The model under review builds one solid part; all positions refer to its coordinate system, in mm. A direction names the side the tool comes from. Give positions to 0.01 mm unless a question says otherwise; leave off trailing zeros. Order: outer loops, then holes, each group sorted by start corner. A loop starts at its lowest first (then second) coordinate and runs counter-clockwise, first axis right, second up. Notation, with made-up numbers: (55, 59) - (88, 59) arc R28 cw to (88, 79) - close; hole circle Ø5 at (-26.5, 32.25). An arc over 180 degrees is marked (long way). Write item = value, one per line. Start each with the question number.
1. Wall thickness on probe 1 along X at (y, z) = (-14, 125.5); probe 2 along X at (y, z) = (4, 54): over which ranges is each line inside the solid? List them lowest first.
2. Mouldability with a two-part tool opening along X and no side actions: class faces 1 (the flat face through (11, -20, 76)), 2 (the cylindrical face through (-18.717, 18.647, 75.922)), 3 (the flat face through (-7.1, -8.6, 75.9)) as pulls with the +X half, pulls with the -X half, needs draft (parallel to the pull), parting line crosses it, or undercut.
3. Machinability: for faces 4 (the flat face through (-5.385, -17, 76)), 5 (the flat face through (5.385, 17, 76)), 6 (the flat face through (17, 2.966, 76)), 7 (the flat face through (-17, 5.266, 76)), which of the approach directions +Z, -Z, +X, -X, +Y, -Y give a long, thin tool a straight path to every point of the face, cutting with its end or side? Answer none if there is none.
4. We need section B-B, the plane x = 1.5. Give the boundary of the cut face in (y, z), and give its area (3 significant figures).
5. For P1, Ø0.5, axis at x = -6, z = 71.5, coming from the -Y side; P2, Ø1.3, axis at x = -17, z = 62, coming from the -Y side; P3, Ø6, axis at x = -3, z = 45, coming from the +Y side; P4, Ø4, axis at x = 15, y = -14, coming from the -Z side, all flat-tipped, find the tip position at first contact; note any pin that passes through.
6. We need section A-A, the plane y = -7. Give the boundary of the cut face in (x, z).
7. We need section C-C, the plane z = 14. State how many separate pieces and enclosed holes the cut face has, and give its area (3 significant figures).
from build123d import *

# Parameters (mm, degrees)
BOSS_EXTRUDE1_DEPTH  = 154
MIRROR3_COPY_1_DEPTH = 154
MIRROR3_COPY_2_DEPTH = 154


with BuildPart() as part:
    # Sketch1 → Boss-Extrude1 (new body)
    with BuildSketch(Plane.XY):
        with BuildLine():
            Line((3.4, 0), (5.5, 0))
            Line((5.5, 0), (5.5, 4))
            Line((5.5, 4), (11.69, 10.19))
            Line((11.69, 10.19), (18.2, 10.19))
            Line((18.2, 10.19), (18.2, 5.265595036))
            Line((18.2, 5.265595036), (15.5, 5.265595036))
            Line((15.5, 5.265595036), (15.5, 2.965595036))
            Line((15.5, 2.965595036), (19, 2.965595036))
            Line((19, 2.965595036), (19, 3.965595036))
            Line((19, 3.965595036), (20, 3.965595036))
            Line((20, 3.965595036), (20, 15.5))
            ThreePointArc((20, 15.5), (18.681980515, 18.681980515), (15.5, 20))
            Line((15.5, 20), (6.385304712, 20))
            Line((6.385304712, 20), (6.385304712, 19))
            Line((6.385304712, 19), (5.385304712, 19))
            Line((5.385304712, 19), (5.385304712, 15.5))
            Line((5.385304712, 15.5), (7.685304712, 15.5))
            Line((7.685304712, 15.5), (7.685304712, 18.2))
            Line((7.685304712, 18.2), (10.19, 18.2))
            Line((10.19, 18.2), (10.19, 11.69))
            Line((10.19, 11.69), (4, 5.5))
            Line((4, 5.5), (0, 5.5))
            Line((0, 5.5), (0, 3.4))
            ThreePointArc((0, 3.4), (2.404163056, 2.404163056), (3.4, 0))
        make_face()
        with BuildLine():
            Line((18.5, 11.69), (18.5, 15.5))
            ThreePointArc((18.5, 15.5), (17.621320344, 17.621320344), (15.5, 18.5))
            Line((15.5, 18.5), (11.69, 18.5))
            Line((11.69, 18.5), (11.69, 11.69))
            Line((11.69, 11.69), (18.5, 11.69))
        make_face(mode=Mode.SUBTRACT)
    boss_extrude1 = extrude(amount=BOSS_EXTRUDE1_DEPTH)

    # Mirror1: Boss-Extrude1 across plane
    add(boss_extrude1.mirror(Plane.ZX))

    # Mirror2: Boss-Extrude1 across plane
    add(boss_extrude1.mirror(Plane(origin=(0, 0, 0), x_dir=(0, 0, 1), z_dir=(1, 0, 0))))

    # Mirror3 copy 1 sketch → Mirror3 copy 1 (add)
    with BuildSketch(Plane(origin=(0, 0, 0), x_dir=(-1, 0, 0), z_dir=(0, 0, 1))):
        with BuildLine():
            Line((3.4, 0), (5.5, 0))
            Line((5.5, 0), (5.5, 4))
            Line((5.5, 4), (11.69, 10.19))
            Line((11.69, 10.19), (18.2, 10.19))
            Line((18.2, 10.19), (18.2, 5.265595036))
            Line((18.2, 5.265595036), (15.5, 5.265595036))
            Line((15.5, 5.265595036), (15.5, 2.965595036))
            Line((15.5, 2.965595036), (19, 2.965595036))
            Line((19, 2.965595036), (19, 3.965595036))
            Line((19, 3.965595036), (20, 3.965595036))
            Line((20, 3.965595036), (20, 15.5))
            ThreePointArc((20, 15.5), (18.681980515, 18.681980515), (15.5, 20))
            Line((15.5, 20), (6.385304712, 20))
            Line((6.385304712, 20), (6.385304712, 19))
            Line((6.385304712, 19), (5.385304712, 19))
            Line((5.385304712, 19), (5.385304712, 15.5))
            Line((5.385304712, 15.5), (7.685304712, 15.5))
            Line((7.685304712, 15.5), (7.685304712, 18.2))
            Line((7.685304712, 18.2), (10.19, 18.2))
            Line((10.19, 18.2), (10.19, 11.69))
            Line((10.19, 11.69), (4, 5.5))
            Line((4, 5.5), (0, 5.5))
            Line((0, 5.5), (0, 3.4))
            ThreePointArc((0, 3.4), (2.404163056, 2.404163056), (3.4, 0))
        make_face()
        with BuildLine():
            Line((18.5, 11.69), (18.5, 15.5))
            ThreePointArc((18.5, 15.5), (17.621320344, 17.621320344), (15.5, 18.5))
            Line((15.5, 18.5), (11.69, 18.5))
            Line((11.69, 18.5), (11.69, 11.69))
            Line((11.69, 11.69), (18.5, 11.69))
        make_face(mode=Mode.SUBTRACT)
    extrude(amount=MIRROR3_COPY_1_DEPTH)

    # Mirror3 copy 2 sketch → Mirror3 copy 2 (add)
    with BuildSketch(Plane.XY):
        with BuildLine():
            Line((3.4, 0), (5.5, 0))
            Line((5.5, 0), (5.5, -4))
            Line((5.5, -4), (11.69, -10.19))
            Line((11.69, -10.19), (18.2, -10.19))
            Line((18.2, -10.19), (18.2, -5.265595036))
            Line((18.2, -5.265595036), (15.5, -5.265595036))
            Line((15.5, -5.265595036), (15.5, -2.965595036))
            Line((15.5, -2.965595036), (19, -2.965595036))
            Line((19, -2.965595036), (19, -3.965595036))
            Line((19, -3.965595036), (20, -3.965595036))
            Line((20, -3.965595036), (20, -15.5))
            ThreePointArc((20, -15.5), (18.681980515, -18.681980515), (15.5, -20))
            Line((15.5, -20), (6.385304712, -20))
            Line((6.385304712, -20), (6.385304712, -19))
            Line((6.385304712, -19), (5.385304712, -19))
            Line((5.385304712, -19), (5.385304712, -15.5))
            Line((5.385304712, -15.5), (7.685304712, -15.5))
            Line((7.685304712, -15.5), (7.685304712, -18.2))
            Line((7.685304712, -18.2), (10.19, -18.2))
            Line((10.19, -18.2), (10.19, -11.69))
            Line((10.19, -11.69), (4, -5.5))
            Line((4, -5.5), (0, -5.5))
            Line((0, -5.5), (0, -3.4))
            ThreePointArc((0, -3.4), (2.404163056, -2.404163056), (3.4, 0))
        make_face()
        with BuildLine():
            Line((18.5, -11.69), (18.5, -15.5))
            ThreePointArc((18.5, -15.5), (17.621320344, -17.621320344), (15.5, -18.5))
            Line((15.5, -18.5), (11.69, -18.5))
            Line((11.69, -18.5), (11.69, -11.69))
            Line((11.69, -11.69), (18.5, -11.69))
        make_face(mode=Mode.SUBTRACT)
    extrude(amount=MIRROR3_COPY_2_DEPTH)


solid = part.part
Model answer:
q1.probe_1 = -20 to -18.5, -11.69 to -10.19, 10.19 to 11.69, 18.5 to 20
q1.probe_2 = -20 to -15.5, -5.5 to 5.5, 15.5 to 20
q2.face_1 = needs draft
q2.face_2 = pulls with the -X half
q2.face_3 = undercut
q3.face_4 = +Z, -Z, -Y
q3.face_5 = +Z, -Z, +Y
q3.face_6 = +Z, -Z, +X
q3.face_7 = +Z, -Z
q4.outline = (-5.5, 0) - (-3.05, 0) - (-3.05, 154) - (-5.5, 154) - close; (3.05, 0) - (5.5, 0) - (5.5, 154) - (3.05, 154) - close
q4.area = 754 mm2
q5.P1 = -19
q5.P2 = -19.92
q5.P3 = 19
q5.P4 = through
q6.outline = (-20, 0) - (-18.2, 0) - (-18.2, 154) - (-20, 154) - close; (-8.5, 0) - (-5.5, 0) - (-5.5, 154) - (-8.5, 154) - close; (5.5, 0) - (8.5, 0) - (8.5, 154) - (5.5, 154) - close; (18.2, 0) - (20, 0) - (20, 154) - (18.2, 154) - close
q7.separate_pieces = 1
q7.enclosed_holes = 5
q7.area = 468 mm2
